Can you work these out from the model? Positions are in its coordinate system, mm. A direction names the side the tool comes from. Round coordinates to 2 decimals unless told otherwise and drop trailing zeros. Order: outer loops, then holes, each group sorted by start corner. A loop starts at its lowest first (then second) coordinate and runs counter-clockwise, first axis right, second up. Notation, with made-up numbers: (-3.75, -10) -> (12.25, -10) arc R33 ccw to (12.25, 25) -> close; hole circle Ø7 at (85.25, 54.5). An arc over 180 degrees is marked (long way). Use a Markdown table: item, result. Add a question column.
Q1. If we section it at A-A on z = 18: List the corners of the cut face in (x, y) for me.
Q2. We'd pull the mould along X, two halves only. Please class faces 1 (the face through (5, 27, 12)), 2 (the face through (0, 25, 12)), 3 (the face through (76.1, 4.7, 25)): +X half, -X half, draft (parallel to the pull), parting line (faces both ways), or undercut.
Q3. For faces 4 (the face through (120, 27, 15)), 5 (the face through (125, 25, 12)), which set-ups out of +Z, -Z, +X, -X, +Y, -Y let a thin tool reach every point of the face, with its end or its side?
Q4. I need wall thicknesses on line 1 along X through (y, z) = (12.5, 18.5); line 2 along Z through (x, y) = (40, 15). Which ranges of each line are inside material? Lowest first, please. Write a range as [from, to].
Q5. I'm going to push flat-ended pins straight in: pin 1 Ø1 at (x, y) = (103.5, 9) entering from +Z; pin 2 Ø5 at (y, z) = (18.5, 10.5) entering from -X; pin 3 Ø5 at (x, z) = (95.5, 21) entering from +Y. Where does each tip first touch, or does it pass through?
Q6. If we section it at C-C on x = 84.5: List the corners of the cut face in (y, z) for me.
```python
from build123d import *

# Parameters (mm, degrees)
F0_W     = 125
F0_H     = 50
F1_DEPTH = 25
F2_T     = -5
F3_SIZE  = 4.99999


# Not quite as in the source:
# - a fillet or chamfer is up to 0.001 mm smaller than in the source, because OpenCascade refuses the exact size


with BuildPart() as f1:
    # F0 (on Top) → F1 (new body)
    with BuildSketch(Plane.XY):
        with Locations((62.5, 25)):
            Rectangle(F0_W, F0_H)
    extrude(amount=F1_DEPTH)

    # F2
    f2_openings = [f1.faces().sort_by_distance(p)[0] for p in [
        (62.5, 25, 25),
        (62.5, 50, 12.5),
    ]]
    offset(amount=F2_T, openings=f2_openings)

    # F3 (size 5 in the source; OpenCascade refuses exactly that, so slightly less here)
    f3_edges = [f1.edges().sort_by_distance(p)[0] for p in [
        (5, 27.5, 25),
    ]]
    chamfer(f3_edges, length=F3_SIZE)


solid = f1.part
```
Answer below:
| question | item | result |
|---|---|---|
| 1 | outline | (0, 0) -> (125, 0) -> (125, 50) -> (120, 50) -> (120, 5) -> (5, 5) -> (5, 50) -> (0, 50) -> close |
| 2 | face 1 | undercut |
| 2 | face 2 | -X half |
| 2 | face 3 | draft |
| 3 | face 4 | +Z, +Y |
| 3 | face 5 | +Z, -Z, +X, +Y, -Y |
| 4 | line 1 | [0, 5], [120, 125] |
| 4 | line 2 | [0, 5] |
| 5 | pin 1 | z = 5 |
| 5 | pin 2 | x = 0 |
| 5 | pin 3 | y = 5 |
| 6 | outline | (0, 0) -> (50, 0) -> (50, 5) -> (5, 5) -> (5, 25) -> (0, 25) -> close |
